Verification items for the finished model (mm, model axes). A direction names the side the tool comes from. Give positions to 0.01 mm unless a question says otherwise; leave off trailing zeros. Write each loop counter-clockwise with the first axis right and the second up, starting at its lowest first coordinate (ties: lowest second). Pieces come first, ordered by that corner, then holes. Notation, with made-up numbers: (15, 38) -> (56, 38) arc R14 cw to (56, 46) -> close; hole circle Ø4 at (6, -22.5). An arc over 180 degrees is marked (long way). Answer as CSV lines item,"result". Start each with the question number.
1) Material ranges on L1, parallel to X at y = -23.75, z = -17; L2, parallel to X at y = -25, z = -15; L3, parallel to Y at x = 165, z = 3.5, recorded low to high.
2) Tool access check on faces 1 (the flat face through (173, -41, 18)), 2 (the cylindrical face through (147.9, -25, 0.4)). Record the directions out of +Z, -Z, +X, -X, +Y, -Y that give a thin tool (end or side, any length) a straight path to the whole face; none if there is none.
3) Sectioned sample at C-C on x = 153. Record the cut outline in (y, z), and give its area (3 significant figures).
4) Sectioned sample at B-B on x = 177.55. Record the cut outline in (y, z).
5) Mould release check, pull along X, two halves, no side actions. Record for faces 3 (the flat face through (164.763, -41.824, 21.371)), 4 (the cylindrical face through (180.235, -23.451, -14.404)), 5 (the flat face through (168, -23, -25)), 6 (the cylindrical face through (183.131, -48.137, 21.451)): released by +X, released by -X, zero draft, split by the parting line, or undercut.
6) Gauge pin test, flat ends, axial feed: pin 1 Ø12 at (x, z) = (179.5, 8) entering from -Y; pin 2 Ø10 at (y, z) = (-27, -5.5) entering from -X; pin 3 Ø8 at (x, z) = (178, 17.5) entering from +Y; pin 4 Ø5 at (x, z) = (157.55, -15) entering from +Y. Record the tip position at first contact, or that the pin passes through.
7) Sectioned sample at D-D on z = 5. Record the cut outline in (x, y).
8) Sectioned sample at A-A on z = -13. Record the cut outline in (x, y).
Autodesk Inventor part; units mm, degrees
ref_plane "YZ Plane" through (0, 0, 0) normal (1, 0, 0) x (0, 1, 0)
ref_plane "XZ Plane" through (0, 0, 0) normal (0, 1, 0) x (-1, 0, 0)
ref_plane "XY Plane" through (0, 0, 0) normal (0, 0, 1) x (1, 0, 0)
sketch "スケッチ1" plane through (0, 0, 0) normal (0, 0, 1) x (1, 0, 0)
  line L0 (0, 0) -> (410.7754, -157.6819) construction
  line L1 (0, 0) -> (440, 0) construction
  line L2 (460, -20) -> (-20, -20)
  line L3 (-20, -20) -> (-20, 20) construction
  line L4 (-20, 20) -> (460, 20) construction
  line L5 (460, 20) -> (460, -20) construction
  line L6 (460, -20) -> (-20, 20) construction
  line L7 (-20, -20) -> (460, 20) construction
  line L8 (-25.839, -11.5042) -> (422.2796, -183.5209) construction
  line L9 (422.2796, -183.5209) -> (436.6144, -146.1776) construction
  line L10 (436.6144, -146.1776) -> (-11.5042, 25.839)
  line L11 (-11.5042, 25.839) -> (-25.839, -11.5042) construction
  line L12 (-25.839, -11.5042) -> (436.6144, -146.1776) construction
  line L13 (422.2796, -183.5209) -> (-11.5042, 25.839) construction
  circle A0 centre (0, 0) radius 150
  circle A1 centre (0, 0) radius 190
  point P0 (220, 0)
  point P1 (205.3877, -78.8409)
  point P2 (183.5622, -49.04)
  point P3 (188.9444, -20)
  point P4 (148.6607, -20)
  point P5 (145.9541, -34.6036)
  dimension "d0" = 159
  dimension "d1" = 440
  dimension "d2" = 440
  dimension "d3" = 40
  dimension "d4" = 480
  dimension "d5" = 480
  dimension "d6" = 40
  dimension "d7" = 20
  dimension "d8" = 300
  dimension "d30" = 40
extrude "押し出し1" add sketch "スケッチ1" along normal mid plane 50 contours A1 L10 A0 L2 picked at (173.5094, -32.9975)
ref_plane "作業平面1" through (148.6607, -27, 25) normal (0, 1, 0) x (1, 0, 0)
sketch "スケッチ2" plane through (148.6607, -27, 25) normal (0, 1, 0) x (1, 0, 0)
  line L0 (-2.7066, 7) -> (40.2837, 7)
  line L1 (40.2837, 7) -> (40.2837, 50)
  line L2 (40.2837, 50) -> (-2.7066, 50)
  line L3 (-2.7066, 50) -> (-2.7066, 7)
  line L4 (40.2837, 0) -> (0, 0)
  line L5 (-2.7066, 50) -> (0, 50)
  line L6 (40.2837, 50) -> (34.9015, 50)
  point P0 (-148.6607, 25)
  dimension "d13" = 7
extrude "押し出し2" cut sketch "スケッチ2" against normal blind 50
fillet "フィレット1" radius 10 1 edges at (167.8109, -27, 18)
fillet "フィレット2" radius 17 1 edges at (168.8026, -20, 25)
fillet "フィレット3" radius 2 2 edges at (183.5622, -49.04, 21.5) (145.9541, -34.6036, 21.2694)
fillet "フィレット4" radius 2 2 edges at (188.5406, -23.5041, -25) (148.1467, -23.5066, -25)
sketch "スケッチ3" plane through (148.6607, -27, 25) normal (0, -1, 0) x (1, 0, 0)
  line L0 (37.3904, -50) -> (-1.1107, -50)
  line L1 (-1.1107, -50) -> (-1.1107, -17)
  point P0 (-148.6607, -25)
  point P1 (8.8893, -40)
  point P2 (0.9221, -50)
  point P3 (-1.1107, -48)
  point P4 (50.415, -50)
  point P5 (28.8893, -40)
  dimension "d20" = 10
  dimension "d21" = 10
  dimension "d29" = 20
hole "穴1" at (157.55, -27, -15) at (177.55, -27, -15) direction (0, 1, 0) diameter 5.5 end through all
properties part number "scara-base28" material "ABS プラスチック"
Ans:
1,L1,"x = 148.11 to 155.66, 159.44 to 175.66, 179.44 to 188.51"
1,L2,"x = 147.9 to 154.8, 160.3 to 174.8, 180.3 to 188.35"
1,L3,"y = -27 to -20"
2,face 1,"-Z, +X, -X, -Y"
2,face 2,"+Z, -Z, -X, +Y"
3,outline,"(-37.31, 18) -> (-37, 18) arc R10 cw to (-27, 8) -> (-27, -25) -> (-20, -25) -> (-20, 8) arc R17 ccw to (-37, 25) -> (-37.31, 25) -> close"
3,area,"382 mm²"
4,outline,"(-46.73, 18) -> (-37, 18) arc R10 cw to (-27, 8) -> (-27, -12.25) -> (-20, -12.25) -> (-20, 8) arc R17 ccw to (-37, 25) -> (-46.73, 25) -> close; (-27, -25) -> (-20, -25) -> (-20, -17.75) -> (-27, -17.75) -> close"
5,face 3,"released by -X"
5,face 4,"undercut"
5,face 5,"zero draft"
5,face 6,"split by the parting line"
6,pin 1,"stops at y = -29"
6,pin 2,"stops at x = 147.55"
6,pin 3,"stops at y = -20.91"
6,pin 4,"passes through"
7,outline,"(147.55, -27) -> (188.07, -27) arc R190 ccw to (188.94, -20) -> (148.66, -20) arc R150 cw to start"
8,outline,"(147.55, -27) -> (155.66, -27) -> (155.66, -20) -> (148.66, -20) arc R150 cw to start; (159.44, -27) -> (175.66, -27) -> (175.66, -20) -> (159.44, -20) -> close; (179.44, -27) -> (188.07, -27) arc R190 ccw to (188.94, -20) -> (179.44, -20) -> close"
